Verification items for the finished model (mm, model axes). Give positions to 0.01 mm unless a question says otherwise; leave off trailing zeros. Write each loop counter-clockwise with the first axis right and the second up, starting at its lowest first coordinate (ties: lowest second). Pieces come first, ordered by that corner, then holes. Notation, with made-up numbers: (70.25, 79.25) -> (103.25, 79.25) arc R21 cw to (103.25, 105.25) -> close; hole circle Ø11 at (-33.75, 77.5). An arc over 180 degrees is marked (long way). Use one line per item in the form item = value. Start each with the question number.
(1) Section check A-A, the plane y = -83.5. Record the cut outline in (x, z).
(2) Depth check by flat-ended pin: pin 1 Ø1 at (y, z) = (-41, 0.5) entering from -X; pin 2 Ø1.5 at (x, z) = (-36, 2) entering from -Y; pin 3 Ø1.5 at (x, z) = (-7, 1) entering from +Y. Enter the tip coordinate at first touch or a pass-through.
(3) Section check D-D, the plane x = -37. Record the cut outline in (y, z), plus the area to 4 significant figures.
(4) Section check C-C, the plane z = 1.4. State how many separate pieces and enclosed holes the cut face has, plus the area to 3 significant figures.
(5) Release check for a two-part mould opening along Y. For faces 1 (the face through (-67.12, -33.73, 1.48)), 2 (the face through (-74.944, -141.415, 1.521)), 3 (the face through (-42, -87, 0)) record: pulls with the +Y half, pulls with the -Y half, needs draft (parallel to the pull), parting line crosses it, or undercut.
(6) Scan lines: L1, parallel to X at y = -83, z = 0.35; L2, parallel to X at y = -86.5, z = 0.65; L3, parallel to Y at x = -21, z = 2.55. Record each from-to range of solid material in increasing order.
(7) Section check B-B, the plane y = -139.5. Record the cut outline in (x, z).
from build123d import *

# Parameters (mm, degrees)
ESQUISSE1_W                     = 141
ESQUISSE1_H                     = 173.5
BOSS_EXTRU_1_DEPTH              = 3
EMPREINTE1_START                = -93.562592566
EMPREINTE1_OUTLINE_W            = 3
EMPREINTE1_OUTLINE_H            = 3
EMPREINTE1_DEPTH                = 40
EMPREINTE1_START_2              = -28.562592566
EMPREINTE1_2_OUTLINE_W          = 3
EMPREINTE1_2_OUTLINE_H          = 3
EMPREINTE1_2_DEPTH              = 40
ESQUISSE2_W                     = 40
ESQUISSE2_H                     = 3
BOSS_EXTRU_2_DEPTH              = 3
EMPREINTE2_START                = -62.5
EMPREINTE2_OUTLINE_W            = 3
EMPREINTE2_OUTLINE_H            = 3
EMPREINTE2_DEPTH                = 50
EMPREINTE2_START_2              = -168
EMPREINTE2_2_OUTLINE_W          = 3
EMPREINTE2_2_OUTLINE_H          = 3
EMPREINTE2_2_DEPTH              = 33
EMPREINTE2_START_3              = -120
EMPREINTE2_3_OUTLINE_W          = 3
EMPREINTE2_3_OUTLINE_H          = 3
EMPREINTE2_3_DEPTH              = 33
D_GAGEMENT_M31_D                = 3.4
DIAM_TRE_DU_PER_AGE_10_0_10_1_D = 10


# Read off the part's stored shape, not the designer's step: Empreinte1, Empreinte2
with BuildPart() as part:
    # Esquisse1 → Boss.-Extru.1 (new body)
    with BuildSketch(Plane.XY):
        with Locations((-41.062592566, -86.75)):
            Rectangle(ESQUISSE1_W, ESQUISSE1_H)
    extrude(amount=BOSS_EXTRU_1_DEPTH)

    # Empreinte1 outline → Empreinte1 (cut)
    with BuildSketch(Plane.YZ.offset(EMPREINTE1_START)):
        with Locations((-1.5, 1.5)):
            Rectangle(EMPREINTE1_OUTLINE_W, EMPREINTE1_OUTLINE_H)
    extrude(amount=EMPREINTE1_DEPTH, mode=Mode.SUBTRACT)

    # Empreinte1 2 outline → Empreinte1 2 (cut)
    with BuildSketch(Plane.YZ.offset(EMPREINTE1_START_2)):
        with Locations((-1.5, 1.5)):
            Rectangle(EMPREINTE1_2_OUTLINE_W, EMPREINTE1_2_OUTLINE_H)
    extrude(amount=EMPREINTE1_2_DEPTH, mode=Mode.SUBTRACT)

    # Esquisse2 → Boss.-Extru.2 (add)
    with BuildSketch(Plane.XZ.offset(173.5)):
        with Locations((-10.562592566, 1.5)):
            Rectangle(ESQUISSE2_W, ESQUISSE2_H)
        with Locations((-71.562592566, 1.5)):
            Rectangle(ESQUISSE2_W, ESQUISSE2_H)
    extrude(amount=BOSS_EXTRU_2_DEPTH)

    # Empreinte2 outline → Empreinte2 (cut)
    with BuildSketch(Plane(origin=(0, 0, 0), x_dir=(1, 0, 0), z_dir=(0, 1, 0)).offset(EMPREINTE2_START)):
        with Locations((27.937407434, -1.5)):
            Rectangle(EMPREINTE2_OUTLINE_W, EMPREINTE2_OUTLINE_H)
        with Locations((-110.062592566, -1.5)):
            Rectangle(EMPREINTE2_OUTLINE_W, EMPREINTE2_OUTLINE_H)
    extrude(amount=EMPREINTE2_DEPTH, mode=Mode.SUBTRACT)

    # Empreinte2 2 outline → Empreinte2 2 (cut)
    with BuildSketch(Plane(origin=(0, 0, 0), x_dir=(1, 0, 0), z_dir=(0, 1, 0)).offset(EMPREINTE2_START_2)):
        with Locations((27.937407434, -1.5)):
            Rectangle(EMPREINTE2_2_OUTLINE_W, EMPREINTE2_2_OUTLINE_H)
        with Locations((-110.062592566, -1.5)):
            Rectangle(EMPREINTE2_2_OUTLINE_W, EMPREINTE2_2_OUTLINE_H)
    extrude(amount=EMPREINTE2_2_DEPTH, mode=Mode.SUBTRACT)

    # Empreinte2 3 outline → Empreinte2 3 (cut)
    with BuildSketch(Plane(origin=(0, 0, 0), x_dir=(1, 0, 0), z_dir=(0, 1, 0)).offset(EMPREINTE2_START_3)):
        with Locations((27.937407434, -1.5)):
            Rectangle(EMPREINTE2_3_OUTLINE_W, EMPREINTE2_3_OUTLINE_H)
        with Locations((-110.062592566, -1.5)):
            Rectangle(EMPREINTE2_3_OUTLINE_W, EMPREINTE2_3_OUTLINE_H)
    extrude(amount=EMPREINTE2_3_DEPTH, mode=Mode.SUBTRACT)

    # Dégagement M31 (through all)
    with Locations(Plane.XY.offset(3)):
        with Locations((-68.372592566, -34.88), (-20.152592566, -28.52), (-68.372592566, -109.76), (-20.152592566, -110.99)):
            Hole(D_GAGEMENT_M31_D / 2)

    # Diamètre du perçage Ø10.0 (10)1 (through all)
    with Locations(Plane(origin=(0, 0, 0), x_dir=(-1, 0, 0), z_dir=(0, 0, -1))):
        with Locations((79.562592566, -139.5), (79.562592566, -83.5), (5.562592566, -83.5)):
            Hole(DIAM_TRE_DU_PER_AGE_10_0_10_1_D / 2)


solid = part.part
Completed:
q1.outline = (-111.56, 0) -> (-84.56, 0) -> (-84.56, 3) -> (-111.56, 3) -> close; (-74.56, 0) -> (-10.56, 0) -> (-10.56, 3) -> (-74.56, 3) -> close; (-0.56, 0) -> (29.44, 0) -> (29.44, 3) -> (-0.56, 3) -> close
q2.pin_1 = -108.56
q2.pin_2 = -173.5
q2.pin_3 = -3
q3.outline = (-173.5, 0) -> (0, 0) -> (0, 3) -> (-173.5, 3) -> close
q3.area = 520.5 mm²
q4.separate_pieces = 1
q4.enclosed_holes = 7
q4.area = 23,500 mm²
q5.face_1 = undercut
q5.face_2 = undercut
q5.face_3 = needs draft
q6.L1 = -111.56 to -84.54, -74.59 to -10.54, -0.59 to 29.44
q6.L2 = -111.56 to -83.56, -75.56 to -9.56, -1.56 to 29.44
q6.L3 = -176.5 to -112.46, -109.52 to -29.99, -27.05 to -3
q7.outline = (-108.56, 0) -> (-84.56, 0) -> (-84.56, 3) -> (-108.56, 3) -> close; (-74.56, 0) -> (26.44, 0) -> (26.44, 3) -> (-74.56, 3) -> close
